from build123d import *

# Parameters (mm, degrees)
SKETCH1_W               = 220
SKETCH1_H               = 300
BOSS_EXTRUDE1_DEPTH     = 70
SKETCH2_R               = 5
SKETCH2_R_2             = 8
CUT_EXTRUDE1_DEPTH      = 221
CHAMFER1_SIZE           = 50
CHAMFER1_SIZE2          = 45.020202215
FILLET1_R               = 5
FILLET2_R               = 10
FILLET3_R               = 50
SKETCH3_W               = 160
SKETCH3_H               = 45
CUT_EXTRUDE2_DEPTH      = 151
CUT_EXTRUDE2_DEPTH_BACK = 151
FILLET4_R               = 2
FILLET5_R               = 2


with BuildPart() as part:
    # Sketch1 → Boss-Extrude1 (new body)
    with BuildSketch(Plane(origin=(0, 0, 0), x_dir=(1, 0, 0), z_dir=(0, 1, 0))):
        Rectangle(SKETCH1_W, SKETCH1_H)
    extrude(amount=BOSS_EXTRUDE1_DEPTH)

    # Sketch2 → Cut-Extrude1 (cut, through all)
    with BuildSketch(Plane.ZY.offset(110)):
        with Locations((-140.194362572, 60.620694634)):
            Circle(SKETCH2_R)
        with Locations((-92.5, 15)):
            Circle(SKETCH2_R_2)
        with Locations((92.5, 15)):
            Circle(SKETCH2_R_2)
        with Locations((140.194362572, 60.620694634)):
            Circle(SKETCH2_R)
    extrude(amount=-CUT_EXTRUDE1_DEPTH, mode=Mode.SUBTRACT)

    # Chamfer1
    chamfer1_edges = [part.edges().sort_by_distance(p)[0] for p in [
        (0, 0, -150),
        (0, 0, 150),
    ]]
    chamfer1_side = [part.faces().sort_by_distance(p)[0] for p in [
        (0, 0, 0),
    ]]
    chamfer(chamfer1_edges, length=CHAMFER1_SIZE, length2=CHAMFER1_SIZE2, reference=chamfer1_side[0])

    # Fillet1
    fillet1_edges = [part.edges().sort_by_distance(p)[0] for p in [
        (0, 70, -150),
        (0, 70, 150),
    ]]
    fillet(fillet1_edges, radius=FILLET1_R)

    # Fillet2
    fillet2_edges = [part.edges().sort_by_distance(p)[0] for p in [
        (0, 45.020202215, 150),
        (0, 45.020202215, -150),
    ]]
    fillet(fillet2_edges, radius=FILLET2_R)

    # Fillet3
    fillet3_edges = [part.edges().sort_by_distance(p)[0] for p in [
        (0, 0, -100),
        (0, 0, 100),
    ]]
    fillet(fillet3_edges, radius=FILLET3_R)

    # Sketch3 → Cut-Extrude2 (cut, two sides)
    with BuildSketch(Plane.XY) as cut_extrude2_sk:
        with Locations((0, 22.5)):
            Rectangle(SKETCH3_W, SKETCH3_H)
    extrude(amount=CUT_EXTRUDE2_DEPTH, mode=Mode.SUBTRACT)
    extrude(cut_extrude2_sk.sketch, amount=-CUT_EXTRUDE2_DEPTH_BACK, mode=Mode.SUBTRACT)

    # Fillet4
    fillet4_edges = [part.edges().sort_by_distance(p)[0] for p in [
        (-80, 3.320978675, 98.725195725),
        (80, 3.320978675, 98.725195725),
        (80, 43.41487437, -147.956463044),
        (80, 27.44189977, -130.477317315),
        (80, 3.320978675, -98.725195725),
        (80, 27.44189977, 130.477317315),
        (80, 43.41487437, 147.956463044),
        (-80, 0, 0),
        (-80, 27.44189977, -130.477317315),
        (-80, 43.41487437, -147.956463044),
        (-80, 3.320978675, -98.725195725),
        (-80, 43.41487437, 147.956463044),
        (-80, 27.44189977, 130.477317315),
        (80, 0, 0),
    ]]
    fillet(fillet4_edges, radius=FILLET4_R)

    # Fillet5
    fillet5_edges = [part.edges().sort_by_distance(p)[0] for p in [
        (-110, 70, 0),
        (110, 70, 0),
        (-110, 57.236244534, 150),
        (-110, 57.236244534, -150),
        (-110, 68.535533906, 148.535533906),
        (-110, 68.535533906, -148.535533906),
        (110, 57.236244534, -150),
        (110, 57.236244534, 150),
        (110, 68.535533906, 148.535533906),
        (110, 68.535533906, -148.535533906),
        (-110, 27.44189977, -130.477317315),
        (-110, 45.405122637, 149.135454576),
        (-110, 45.405122637, -149.135454576),
        (110, 27.44189977, 130.477317315),
        (110, 45.405122637, 149.135454576),
        (110, 45.405122637, -149.135454576),
        (110, 0, 0),
        (-110, 0, 0),
        (110, 27.44189977, -130.477317315),
        (110, 3.320978675, 98.725195725),
        (110, 3.320978675, -98.725195725),
        (-110, 27.44189977, 130.477317315),
        (-110, 3.320978675, 98.725195725),
        (-110, 3.320978675, -98.725195725),
    ]]
    fillet(fillet5_edges, radius=FILLET5_R)


solid = part.part
Part model, mm, in its own coordinate system. A direction names the side the tool comes from. Give positions to 0.01 mm unless a question says otherwise; leave off trailing zeros. Order: outer loops, then holes, each group sorted by start corner. A loop starts at its lowest first (then second) coordinate and runs counter-clockwise, first axis right, second up. Notation, with made-up numbers: (-29.5, 78.5) - (28.5, 78.5) arc R21 ccw to (28.5, 103.5) - close; hole circle Ø6 at (-14.75, -22). An arc over 180 degrees is marked (long way). Use a Markdown table: item, result.
1) Probe L1, parallel to X at y = 8.5, z = 76.5; L2, parallel to Z at x = 87, y = 9.5; L3, parallel to Y at x = 32.5, z = 82. List the from-to ranges inside material, lowest first. Write a range as from..to.
Checked values:
| item | result |
|---|---|
| L1 | -110..-80, 80..110 |
| L2 | -110.13..-98.31, -86.69..86.69, 98.31..110.13 |
| L3 | 45..70 |
2) Flat gauge pins, fed straight in: P1, Ø14.5, axis at y = 15, z = -92.5, coming from the -X side; P2, Ø13, axis at y = 60.62, z = 140.19, coming from the +X side; P3, Ø8, axis at x = 86.5, z = 117, coming from the -Y side; P4, Ø12, axis at x = -66, z = 71, coming from the -Y side. Where does each tip first touch, or does it go through?
Checked values:
| item | result |
|---|---|
| P1 | through |
| P2 | x = 110 |
| P3 | y = 11.74 |
| P4 | y = 45 |
3) Saw through at A-A on z = -67. List the corners of the cut face in (x, y), plus the area to 3 significant figures.
Checked values:
| item | result |
|---|---|
| outline | (-110, 2) arc R2 ccw to (-108, 0) - (-82, 0) arc R2 ccw to (-80, 2) - (-80, 45) - (80, 45) - (80, 2) arc R2 ccw to (82, 0) - (108, 0) arc R2 ccw to (110, 2) - (110, 68) arc R2 ccw to (108, 70) - (-108, 70) arc R2 ccw to (-110, 68) - close |
| area | 8,190 mm² |
4) Two-plate mould, pull along X, no slides. Class faces 3 (the cylindrical face through (-109.43, 27.684, -129.848)), 4 (the flat face through (95, 0, -1)), 5 (the flat face through (-1, 45, -2)), 6 (the cylindrical face through (80.57, 28.09, -130.3)): +X half, -X half, draft (parallel to the pull), parting line (faces both ways), or undercut.
Checked values:
| item | result |
|---|---|
| face 3 | -X half |
| face 4 | draft |
| face 5 | undercut |
| face 6 | undercut |
5) 3-axis set-ups, long thin cutter, end or side, ignore diameter. For faces 1 (the cylindrical face through (-1.54, 62.123, -135.425)), 2 (the cylindrical face through (-80.57, 27.684, 129.848)): which of +Z, -Z, +X, -X, +Y, -Y reach the whole face in a straight line?
Checked values:
| item | result |
|---|---|
| face 1 | +X, -X |
| face 2 | +Z, -Y |
6) Saw through at B-B on x = 32.5. List the corners of the cut face in (y, z), plus the area to 3 significant figures.
Checked values:
| item | result |
|---|---|
| outline | (45, -148.94) arc R10 ccw to (49.47, -150) - (65, -150) arc R5 ccw to (70, -145) - (70, 145) arc R5 ccw to (65, 150) - (49.47, 150) arc R10 ccw to (45, 148.94) - close; hole circle Ø10 at (60.62, -140.19); hole circle Ø10 at (60.62, 140.19) |
| area | 7,330 mm² |
7) Saw through at C-C on y = 18.5. Count the separate pieces of the cut face and the enclosed holes in it, plus the area to 3 significant figures.
Checked values:
| item | result |
|---|---|
| separate pieces | 6 |
| enclosed holes | 0 |
| area | 12,700 mm² |
